Verification items for the finished model (mm, model axes). A direction names the side the tool comes from. Coordinates: 2 decimals unless noted, no trailing zeros. Order: outer loops, then holes, each group sorted by start corner. A loop starts at its lowest first (then second) coordinate and runs counter-clockwise, first axis right, second up. Notation, with made-up numbers: (-8, -34) -> (28, -34) arc R13 ccw to (28, -19) -> close; hole circle Ø3 at (-24.75, -9). An arc over 180 degrees is marked (long way). Use CSV: the item, a comma, the result in double quotes. Start each with the question number.
1) Sectioned sample at D-D on z = -2.25. Record the boundary of the cut face in (x, y), then the cut area to 3 significant figures.
2) Sectioned sample at B-B on y = -30. Record the boundary of the cut face in (x, z).
3) Tool access check on faces 5 (the cylindrical face through (22.4, -30.39, 9.43)), 6 (the flat face through (15, -30, -5)). Record the directions out of +Z, -Z, +X, -X, +Y, -Y that give a thin tool (end or side, any length) a straight path to the whole face; none if there is none.
4) Scan lines: line 1 along Y through (x, z) = (0, 7.5); line 2 along X through (y, z) = (-25.5, -2); line 3 along Z through (x, y) = (-3, -12). Record each from-to range of solid material in increasing order.
5) Go/stop test with flat-tipped pins: pin 1 (15 mm diameter, centred on x = -7, y = -29, fed in from -Z); pin 2 (15.5 mm diameter, centred on x = 0, y = -30, fed in from +Z). Record where each tip stops, or that it passes through.
6) Release check for a two-part mould opening along X. For faces 1 (the flat face through (-7, -30, 0)), 2 (the flat face through (-15, -30, -5)), 3 (the cylindrical face through (-22.43, -59.4, -1.13)), 4 (the flat face through (-19, -30, -10)) record: released by +X, released by -X, zero draft, split by the parting line, or undercut.
7) Sectioned sample at C-C on z = 3. Record the boundary of the cut face in (x, y), then the cut area to 3 significant figures.
8) Sectioned sample at A-A on x = 0. Record the boundary of the cut face in (y, z).
from build123d import *

# Parameters (mm, degrees)
F1_DEPTH = 60
F2_R     = 6
F3_DEPTH = 25
F4_R     = 2


with BuildPart() as f1:
    # F0 (on Front) → F1 (new body)
    with BuildSketch(Plane.XZ):
        Polygon((-23, 10), (-23, -10), (-15, -10), (-15, 0), (15, 0), (15, -10), (23, -10), (23, 10), align=None)
    extrude(amount=F1_DEPTH)

    # F2 (on face) → F3 (cut)
    with BuildSketch(Plane.XY.offset(10)):
        with Locations((0, -30)):
            Circle(F2_R)
    extrude(amount=-F3_DEPTH, mode=Mode.SUBTRACT)

    # F4
    f4_edges = [f1.edges().sort_by_distance(p)[0] for p in [
        (0, 0, 10),
        (23, 0, 0),
        (-23, 0, 0),
        (-23, -60, 0),
        (-23, -30, 10),
        (0, -60, 10),
        (23, -30, 10),
        (23, -60, 0),
    ]]
    fillet(f4_edges, radius=F4_R)


solid = f1.part
Answers follow:
1,outline,"(-23, -58) arc R2 ccw to (-21, -60) -> (-15, -60) -> (-15, 0) -> (-21, 0) arc R2 ccw to (-23, -2) -> close; (15, -60) -> (21, -60) arc R2 ccw to (23, -58) -> (23, -2) arc R2 ccw to (21, 0) -> (15, 0) -> close"
1,area,"957 mm²"
2,outline,"(-23, -10) -> (-15, -10) -> (-15, 0) -> (-6, 0) -> (-6, 10) -> (-21, 10) arc R2 ccw to (-23, 8) -> close; (6, 0) -> (15, 0) -> (15, -10) -> (23, -10) -> (23, 8) arc R2 ccw to (21, 10) -> (6, 10) -> close"
3,face 5,"+Z, +X, +Y, -Y"
3,face 6,"-Z, +Y, -Y"
4,line 1,"y = -60 to -36, -24 to 0"
4,line 2,"x = -23 to -15, 15 to 23"
4,line 3,"z = 0 to 10"
5,pin 1,"stops at z = 0"
5,pin 2,"stops at z = 10"
6,face 1,"undercut"
6,face 2,"undercut"
6,face 3,"released by -X"
6,face 4,"zero draft"
7,outline,"(-23, -58) arc R2 ccw to (-21, -60) -> (21, -60) arc R2 ccw to (23, -58) -> (23, -2) arc R2 ccw to (21, 0) -> (-21, 0) arc R2 ccw to (-23, -2) -> close; hole circle Ø12 at (0, -30)"
7,area,"2,640 mm²"
8,outline,"(-60, 0) -> (-36, 0) -> (-36, 10) -> (-58, 10) arc R2 ccw to (-60, 8) -> close; (-24, 0) -> (0, 0) -> (0, 8) arc R2 ccw to (-2, 10) -> (-24, 10) -> close"
